Part model, mm, in its own coordinate system. A direction names the side the tool comes from. Coordinates: 2 decimals unless noted, no trailing zeros. Order: outer loops, then holes, each group sorted by start corner. A loop starts at its lowest first (then second) coordinate and runs counter-clockwise, first axis right, second up. Notation, with made-up numbers: (-7.5, -26.75) - (17.5, -26.75) arc R18 ccw to (17.5, -17.75) - close; hole circle Ø5 at (66.5, 42.5). An arc over 180 degrees is marked (long way). Use a Markdown table: item, result. Add a question column.
1) Tool access for faces 5 (the face through (24, -21, 0)), 6 (the face through (31.4, -23.05, 8.4)), 7 (the face through (30.885, -21, 15)): list every direction of +Z, -Z, +X, -X, +Y, -Y with a clear straight run to the whole face (end or side of a thin tool).
2) Saw through at A-A on z = 19. List the corners of the cut face in (x, y).
3) Saw through at D-D on z = 10.5. List the corners of the cut face in (x, y), then the cut area to 3 significant figures.
4) Drop flat-ended pins along their axis: P1, Ø0.8, axis at x = 31.5, y = -22, coming from the -Z side; P2, Ø3.5, axis at x = 18.78, y = -20.36, coming from the +Z side; P3, Ø2, axis at y = -19.5, z = 15.5, coming from the -X side; P4, Ø2, axis at y = -21.5, z = 9.5, coming from the -X side. Give the stop position or say it passes through.
5) Saw through at B-B on x = 28. List the corners of the cut face in (y, z), then the cut area to 3 significant figures.
6) Two-plate mould, pull along X, no slides. Class faces 1 (the face through (14.385, -21, 1)), 2 (the face through (31.3, -17.759, 6.3)), 3 (the face through (17.08, -21.67, 1.48)), 4 (the face through (30.754, -21.58, 1.479)): +X half, -X half, draft (parallel to the pull), parting line (faces both ways), or undercut.
7) Wall check: L1, parallel to Y at x = 29, z = 1.25; L2, parallel to X at y = -19.75, z = 2.25; L3, parallel to X at y = -18.5, z = 8.5. Give the ranges that are in metal, low to high. Write a range as [from, to].
8) Saw through at C-C on y = -21.75. List the corners of the cut face in (x, z), then the cut area to 3 significant figures.
```python
from build123d import *

# Parameters (mm, degrees)
SKETCH1_W               = 19.5
SKETCH1_H               = 6.5
BOSS_EXTRUDE1_DEPTH     = 3
SKETCH2_W               = 3
SKETCH2_H               = 6.5
BOSS_EXTRUDE2_DEPTH     = 20
SKETCH3_R               = 1.5
CUT_EXTRUDE1_DEPTH      = 10
CUT_EXTRUDE2_DEPTH      = 10
CUT_EXTRUDE2_DEPTH_BACK = 10
SKETCH4_R               = 2.15
SKETCH5_W               = 10.88141253
SKETCH5_H               = 4.494582939
CUT_EXTRUDE3_DEPTH      = 1


with BuildPart() as part:
    # Sketch1 → Boss-Extrude1 (new body)
    with BuildSketch(Plane.XY):
        with Locations((24.134573854, -21.008812853)):
            Rectangle(SKETCH1_W, SKETCH1_H)
    extrude(amount=BOSS_EXTRUDE1_DEPTH)

    # Sketch2 → Boss-Extrude2 (add)
    with BuildSketch(Plane.XY.offset(3)):
        with Locations((32.384573854, -21.008812853)):
            Rectangle(SKETCH2_W, SKETCH2_H)
    extrude(amount=BOSS_EXTRUDE2_DEPTH)

    # Sketch3 → Cut-Extrude1 (cut)
    with BuildSketch(Plane.ZY.offset(-30.884573854)):
        with Locations(Location((19, -21.258812853, 0), (0, 0, 270))):
            Circle(SKETCH3_R)
    extrude(amount=-CUT_EXTRUDE1_DEPTH, mode=Mode.SUBTRACT)

    # Sketch4 → Cut-Extrude2 (cut, two sides: drawn at the far end of the back side and taken through both)
    with BuildSketch(Plane.XY.offset(3).offset(-CUT_EXTRUDE2_DEPTH_BACK)):
        with Locations(Location((28.984573854, -20.358812853, 0), (0, 0, 27.905472791))):
            Circle(SKETCH4_R)
        with Locations((18.784573854, -20.358812853)):
            Circle(SKETCH4_R)
    extrude(amount=CUT_EXTRUDE2_DEPTH + CUT_EXTRUDE2_DEPTH_BACK, mode=Mode.SUBTRACT)

    # Sketch5 → Cut-Extrude3 (cut)
    with BuildSketch(Plane.ZY.offset(-30.884573854)):
        with Locations((8.440706265, -20.802989028)):
            Rectangle(SKETCH5_W, SKETCH5_H)
    extrude(amount=-CUT_EXTRUDE3_DEPTH, mode=Mode.SUBTRACT)


solid = part.part
```
Results are:
| question | item | result |
|---|---|---|
| 1 | face 5 | -Z, +X, -X, +Y, -Y |
| 1 | face 6 | -X |
| 1 | face 7 | +Z, -X, +Y, -Y |
| 2 | outline | (30.88, -24.26) - (33.88, -24.26) - (33.88, -22.76) - (30.88, -22.76) - close; (30.88, -19.76) - (33.88, -19.76) - (33.88, -17.76) - (30.88, -17.76) - close |
| 3 | outline | (30.88, -24.26) - (33.88, -24.26) - (33.88, -17.76) - (30.88, -17.76) - (30.88, -18.56) - (31.88, -18.56) - (31.88, -23.05) - (30.88, -23.05) - close |
| 3 | area | 15.0 mm2 |
| 4 | P1 | z = 0 |
| 4 | P2 | through |
| 4 | P3 | x = 30.88 |
| 4 | P4 | x = 31.88 |
| 5 | outline | (-24.26, 0) - (-22.27, 0) - (-22.27, 3) - (-24.26, 3) - close; (-18.45, 0) - (-17.76, 0) - (-17.76, 3) - (-18.45, 3) - close |
| 5 | area | 8.03 mm2 |
| 6 | face 1 | -X half |
| 6 | face 2 | draft |
| 6 | face 3 | undercut |
| 6 | face 4 | undercut |
| 7 | L1 | [-24.26, -22.51], [-18.21, -17.76] |
| 7 | L2 | [14.38, 16.72], [20.85, 26.92], [31.05, 33.88] |
| 7 | L3 | [30.88, 33.88] |
| 8 | outline | (14.38, 0) - (17.15, 0) - (17.15, 3) - (14.38, 3) - close; (20.42, 0) - (27.35, 0) - (27.35, 3) - (20.42, 3) - close; (30.62, 0) - (33.88, 0) - (33.88, 17.58) - (30.88, 17.58) - (30.88, 13.88) - (31.88, 13.88) - (31.88, 3) - (30.62, 3) - close; (30.88, 20.42) - (33.88, 20.42) - (33.88, 23) - (30.88, 23) - close |
| 8 | area | 79.4 mm2 |
